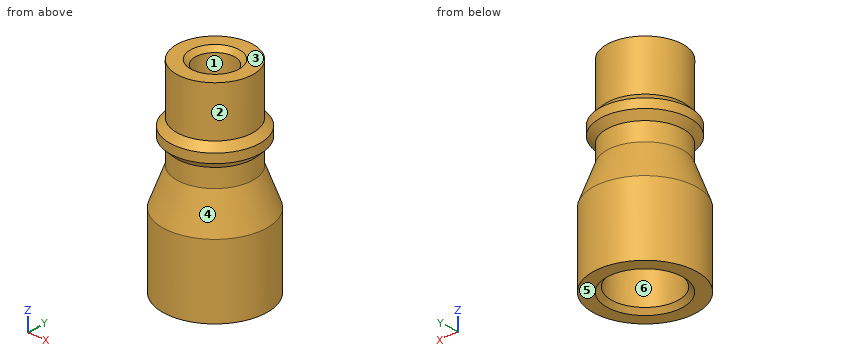
from build123d import *

# Parameters (mm, degrees)
SKETCH1_R           = 5.65
SKETCH1_R_2         = 3.65
BOSS_EXTRUDE1_DEPTH = 8
SKETCH3_R           = 5.65
SKETCH2_R           = 4.15
SKETCH4_R           = 3.65
CUT_EXTRUDE2_DEPTH  = 3
CUT_EXTRUDE2_TAPER  = 49
SKETCH6_R           = 4.15
SKETCH6_R_2         = 2.15
BOSS_EXTRUDE2_DEPTH = 10
CHAMFER1_SIZE       = 0.5
CHAMFER2_SIZE       = 0.5


with BuildPart() as part:
    # Sketch1 → Boss-Extrude1 (new body)
    with BuildSketch(Plane.XY):
        Circle(SKETCH1_R)
        Circle(SKETCH1_R_2, mode=Mode.SUBTRACT)
    extrude(amount=BOSS_EXTRUDE1_DEPTH)

    # Sketch3 → Loft1 section 0
    with BuildSketch(Plane.XY.offset(8)):
        Circle(SKETCH3_R)
    # Sketch2 → Loft1 section 1
    with BuildSketch(Plane.XY.offset(12)):
        Circle(SKETCH2_R)
    loft()

    # Sketch4 → Cut-Extrude2 (cut)
    with BuildSketch(Plane(origin=(0, 0, 8), x_dir=(-1, 0, 0), z_dir=(0, 0, -1))):
        Circle(SKETCH4_R)
    extrude(amount=-CUT_EXTRUDE2_DEPTH, taper=CUT_EXTRUDE2_TAPER, mode=Mode.SUBTRACT)

    # Sketch6 → Boss-Extrude2 (add)
    with BuildSketch(Plane.XY.offset(12)):
        Circle(SKETCH6_R)
        Circle(SKETCH6_R_2, mode=Mode.SUBTRACT)
    extrude(amount=BOSS_EXTRUDE2_DEPTH)

    # Sketch7 → Revolve1 (revolve)
    with BuildSketch(Plane(origin=(0, 0, 0), x_dir=(0, 0, -1), z_dir=(1, 0, 0))):
        Polygon((-14, 4.15), (-14.75, 4.9), (-15.75, 4.9), (-16.5, 4.15), align=None)
    revolve(axis=Axis((0, 0, -80.9), (0, 0, 1)))

    # Chamfer1
    chamfer1_edges = [part.edges().sort_by_distance(p)[0] for p in [
        (-3.65, 0, 0),
    ]]
    chamfer(chamfer1_edges, length=CHAMFER1_SIZE)

    # Chamfer2
    chamfer2_edges = [part.edges().sort_by_distance(p)[0] for p in [
        (-2.15, 0, 22),
    ]]
    chamfer(chamfer2_edges, length=CHAMFER2_SIZE)


solid = part.part
Work out the finished part from the listing and answer in its coordinate system (mm). Face numbers are marked on the shaded views. A direction names the side the tool comes from. Round coordinates to 2 decimals unless told otherwise and drop trailing zeros. Write each loop counter-clockwise with the first axis right and the second up, starting at its lowest first coordinate (ties: lowest second). Pieces come first, ordered by that corner, then holes. Notation, with made-up numbers: (0.5, -19) - (18.5, -19) arc R18 cw to (18.5, -15) - close; hole circle Ø2 at (-40, 59). An arc over 180 degrees is marked (long way). Answer in a Markdown table with one row per item. Add a question column.
1. A cutting plane is placed at A-A, the plane z = 12.25. Determine the outline of the cut face in (x, y), and give its area (3 significant figures).
2. Find the intervals of material crossed by line 1 along Y through (x, z) = (0, 2.75); line 2 along Y through (x, z) = (0, 15.25); line 3 along X through (y, z) = (-1.25, 1), in increasing order. Write a range as from..to.
3. The mould has two halves that part along Y. Classify the marked faces 1, 2 and 3: +Y half, -Y half, draft (parallel to the pull), parting line (faces both ways), or undercut.
4. For the marked faces 4, 5 and 6, determine the directions among +Z, -Z, +X, -X, +Y, -Y from which every point of the face is accessible in a straight line to the end or side of a thin tool.
5. Given pin 1 (1 mm diameter, centred on x = -2, y = -4, fed in from -Z); pin 2 (1.5 mm diameter, centred on x = 3.5, y = -4, fed in from +Z); pin 3 (5 mm diameter, centred on x = 0, y = 0, fed in from -Z); pin 4 (2 mm diameter, centred on x = -1, y = 0.5, fed in from +Z), each flat-ended and moving along its own axis, determine where each tip first touches the part or whether it passes through.
6. A cutting plane is placed at B-B, the plane z = 6.75. Determine the outline of the cut face in (x, y), and give its area (3 significant figures).
Worked out:
| question | item | result |
|---|---|---|
| 1 | outline | circle Ø8.3 at (0, 0); hole circle Ø4.3 at (0, 0) |
| 1 | area | 39.6 mm^2 |
| 2 | line 1 | -5.65..-3.65, 3.65..5.65 |
| 2 | line 2 | -4.9..-2.15, 2.15..4.9 |
| 2 | line 3 | -5.51..-3.43, 3.43..5.51 |
| 3 | face 1 | undercut |
| 3 | face 2 | parting line |
| 3 | face 3 | draft |
| 4 | face 4 | none |
| 4 | face 5 | -Z, +X, -X, +Y, -Y |
| 4 | face 6 | -Z |
| 5 | pin 1 | z = 0 |
| 5 | pin 2 | z = 16.08 |
| 5 | pin 3 | z = 9 |
| 5 | pin 4 | z = 12 |
| 6 | outline | circle Ø11.3 at (0, 0); hole circle Ø7.3 at (0, 0) |
| 6 | area | 58.4 mm^2 |
